Can you work these out from the drawing? Everything is in mm from the part's minimum corner. A direction names the side the tool comes from. Round coordinates to 2 decimals unless told otherwise and drop trailing zeros. Write each loop counter-clockwise with the first axis right and the second up, starting at its lowest first coordinate (ties: lowest second). Pieces come first, ordered by that corner, then holes. Notation, with made-up numbers: (70, 74.5) - (94, 74.5) arc R25 cw to (94, 89.5) - close; hole circle Ø9 at (71.25, -7.5). An arc over 180 degrees is marked (long way). Write each question's results on one line, items separated by ' | '. Start each with the question number.
(1) For P1, Ø9, axis at x = 8.5, y = 27.5, coming from the -Z side; P2, Ø2.5, axis at x = 8, z = 8, coming from the -Y side; P3, Ø1.5, axis at y = 41, z = 7, coming from the +X side, each with a flat end and sliding along its axis, tell me the tip position at first contact or that it passes through.
(2) Imagine slicing it at B-B on y = 10. Write out the boundary of the cut face in (x, z).
(3) Imagine slicing it at A-A on z = 6.25. Write out the boundary of the cut face in (x, y).
(4) On a 3-axis mill with a long thin cutter (end or side, diameter ignored), from which of +Z, -Z, +X, -X, +Y, -Y can I reach the whole of each face in a straight line? I mean the marked faces 1, 2, 3, 4 and 5. Say none if no direction works.
(5) Imagine slicing it at C-C on x = 12. Write out the boundary of the cut face in (y, z).
(6) Imagine slicing it at D-D on z = 10.75. Write out the boundary of the cut face in (x, y), then the cut area to 3 significant figures.
(7) Please list where these lines run through material, in increasing order: line 1 (Z direction, x = 19, y = 6); line 2 (Y direction, x = 9, z = 6); line 3 (X direction, y = 57, z = 8.75). Write a range as [from, to].
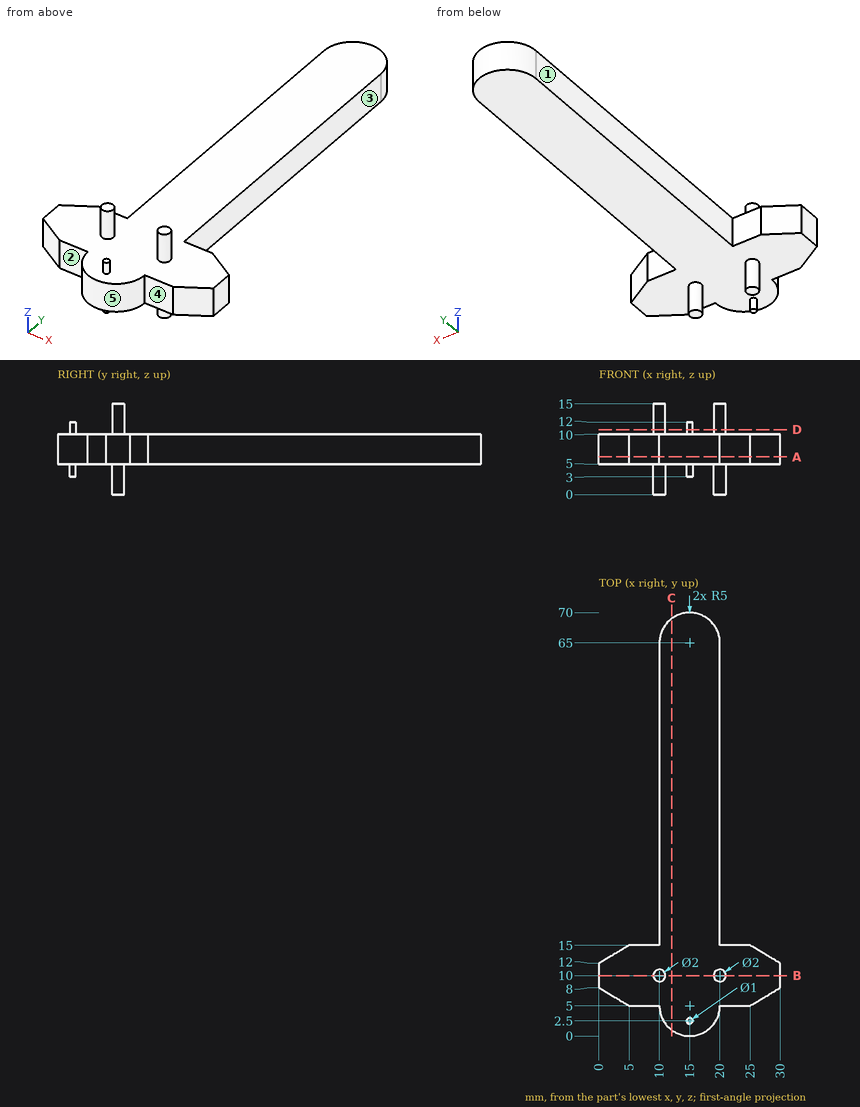
Response:
1) P1: z = 5 | P2: y = 5 | P3: x = 20
2) outline: (0, 5) - (9, 5) - (9, 0) - (11, 0) - (11, 5) - (19, 5) - (19, 0) - (21, 0) - (21, 5) - (30, 5) - (30, 10) - (21, 10) - (21, 15) - (19, 15) - (19, 10) - (11, 10) - (11, 15) - (9, 15) - (9, 10) - (0, 10) - close
3) outline: (0, 8) - (5, 5) - (10, 5) arc R5 ccw to (20, 5) - (25, 5) - (30, 8) - (30, 12) - (25, 15) - (20, 15) - (20, 65) arc R5 ccw to (10, 65) - (10, 15) - (5, 15) - (0, 12) - close
4) face 1: +Z, -Z, -X, +Y | face 2: +Z, -Z, -X, -Y | face 3: +Z, -Z, +X, +Y | face 4: +Z, -Z, +X, -Y | face 5: +Z, -Z, -Y
5) outline: (1, 5) - (69, 5) - (69, 10) - (1, 10) - close
6) outline: circle Ø2 at (10, 10); circle Ø1 at (15, 2.5); circle Ø2 at (20, 10) | area: 7.07 mm²
7) line 1: [5, 10] | line 2: [5, 15] | line 3: [10, 20]
